from build123d import *

# Parameters (mm, degrees)
EXTRUIR_L_MINA1_DEPTH = 25.4
CROQUIS2_R            = 4.7625
CORTAR_EXTRUIR1_DEPTH = 56.634162167


with BuildPart() as part:
    # Croquis1 → Extruir-Lámina1 (new, symmetric)
    with BuildSketch(Plane.XY):
        Polygon((0, 0), (25, 0), (25, 35), (35, 35), (35, 45), (15, 45), (15, 10), (0, 10), align=None)
    extrude(amount=EXTRUIR_L_MINA1_DEPTH, both=True)

    # Croquis2 → Cortar-Extruir1 (cut, through all)
    with BuildSketch(Plane(origin=(0, 10, 0), x_dir=(1, 0, 0), z_dir=(0, 1, 0))):
        with Locations(Location((7.5, 0, 0), (0, 0, 270))):
            Circle(CROQUIS2_R)
    extrude(amount=-CORTAR_EXTRUIR1_DEPTH, mode=Mode.SUBTRACT)


solid = part.part
Can you work these out from the model? Positions are in its coordinate system, mm. A direction names the side the tool comes from. Coordinates: 2 decimals unless noted, no trailing zeros. Write each loop counter-clockwise with the first axis right and the second up, starting at its lowest first coordinate (ties: lowest second). Pieces come first, ordered by that corner, then holes. Notation, with made-up numbers: (46.5, 16) - (85.5, 16) arc R15 cw to (85.5, 22) - close; hole circle Ø2 at (-23, 79.5). An arc over 180 degrees is marked (long way). Return JSON: item names as keys, results as strings. Group by question number.
Item 1: We'd pull the mould along Z, two halves only. Please class faces 1 (the face through (12.22, 5.07, -0.62)), 2 (the face through (25, 17, 0)), 3 (the face through (17, 23, 25.4)), 4 (the face through (17, 23, -25.4)): pulls with the +Z half, pulls with the -Z half, needs draft (parallel to the pull), parting line crosses it, or undercut.
Item 2: If we section it at A-A (x = 7.5): Write out the boundary of the cut face in (y, z), then the cut area to 3 significant figures.
Item 3: Please list where these lines run through material, in increasing order: probe 1 along X at (y, z) = (5.25, 0); probe 2 along Y at (x, z) = (28.5, -10.5); probe 3 along X at (y, z) = (27.5, 8).
Item 4: Which directions (+Z, -Z, +X, -X, +Y, -Y) give clear straight access to the entire face, cutting with the end or side of a thin tool? Please do faces 5 (the face through (25, 45, 0)), 6 (the face through (30, 35, 0)), 7 (the face through (15, 28, 0)).
Item 5: I'm going to push flat-ended pins straight in: pin 1 Ø17.5 at (y, z) = (25.5, -10) entering from +X; pin 2 Ø12 at (y, z) = (40.5, -19) entering from -X; pin 3 Ø5 at (x, z) = (30.5, 12.5) entering from -Y. Where does each tip first touch, or does it pass through?
Item 6: If we section it at D-D (y = 42): Write out the boundary of the cut face in (x, z).
Item 7: If we section it at C-C (z = -7): Write out the boundary of the cut face in (x, y).
Item 8: If we section it at B-B (z = 0): Write out the boundary of the cut face in (x, y), then the cut area to 3 significant figures.
Return value:
{
 "1": {"face 1": "undercut", "face 2": "needs draft", "face 3": "pulls with the +Z half", "face 4": "pulls with the -Z half"},
 "2": {"outline": "(0, -25.4) - (10, -25.4) - (10, -4.76) - (0, -4.76) - close; (0, 4.76) - (10, 4.76) - (10, 25.4) - (0, 25.4) - close", "area": "413 mm^2"},
 "3": {"probe 1": "x = 0 to 2.74, 12.26 to 25", "probe 2": "y = 35 to 45", "probe 3": "x = 15 to 25"},
 "4": {"face 5": "+Z, -Z, +X, -X, +Y", "face 6": "+Z, -Z, +X, -Y", "face 7": "+Z, -Z, -X, +Y"},
 "5": {"pin 1": "stops at x = 25", "pin 2": "stops at x = 15", "pin 3": "stops at y = 35"},
 "6": {"outline": "(15, -25.4) - (35, -25.4) - (35, 25.4) - (15, 25.4) - close"},
 "7": {"outline": "(0, 0) - (25, 0) - (25, 35) - (35, 35) - (35, 45) - (15, 45) - (15, 10) - (0, 10) - close"},
 "8": {"outline": "(0, 0) - (2.74, 0) - (2.74, 10) - (0, 10) - close; (12.26, 0) - (25, 0) - (25, 35) - (35, 35) - (35, 45) - (15, 45) - (15, 10) - (12.26, 10) - close", "area": "605 mm^2"}
}
